For this review, take the finished solid that the model builds, in its own axes (mm). Face numbers are marked on the shaded views. A direction names the side the tool comes from. Round coordinates to 2 decimals unless told otherwise and drop trailing zeros. Loops run counter-clockwise (first coordinate to the right, second up) from the corner with the lowest first, then second, coordinate; pieces in that order, holes last.
1. To check wall thickness, follow line 1 along Z through (x, y) = (25.45, 0); line 2 along X through (y, z) = (7.75, 17.5); line 3 along Z through (x, y) = (0.5, 8.5). State the ranges of each line that lie inside material, in increasing order.
2. Consider section C-C on y = 10. State the section outline as (x, z) points, then the cut area to 3 significant figures.
3. Tool access review of the marked faces 1, 2 and 3: name each direction out of +Z, -Z, +X, -X, +Y, -Y from which nothing blocks a thin tool from reaching the whole face with its end or side.
4. Consider section D-D on y = -7.25. State the section outline as (x, z) points, then the cut area to 3 significant figures.
5. Clearance check with flat-ended pins moving along their axes: pin 1 Ø1.2 at (y, z) = (14, 10) entering from +X; pin 2 Ø4 at (y, z) = (3, 5) entering from -X; pin 3 Ø4 at (x, y) = (-2.5, 8.5) entering from +Z. State where each tip first meets the part, or that it passes through.
6. Consider section B-B on z = 3. State the section outline as (x, y) points, then the cut area to 3 significant figures.
7. Consider section A-A on y = 0. State the section outline as (x, z) points, then the cut area to 3 significant figures.
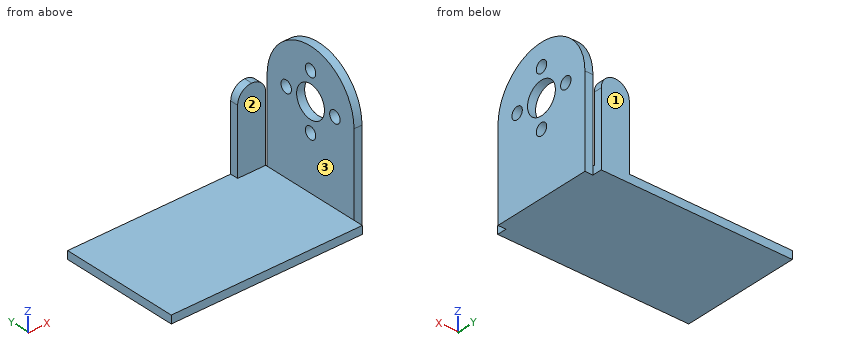
from build123d import *

# Parameters (mm, degrees)
SKETCH_1_W          = 47.7
SKETCH_1_H          = 29.8
EXTRUDE_1_DEPTH     = 2
SKETCH_2_W          = 7
SKETCH_2_H          = 2
EXTRUDE_3_DEPTH     = 19.9
CUT_EXTRUDE_1_DEPTH = 43.676369339
SKETCH_4_R          = 4
SKETCH_4_R_2        = 1.5
EXTRUDE_4_DEPTH     = 2
SKETCH_5_R          = 4
SKETCH_5_R_2        = 1.5
EXTRUDE_5_DEPTH     = 2


with BuildPart() as part:
    # 스케치1 → 보스-돌출1 (new body)
    with BuildSketch(Plane.XY):
        Rectangle(SKETCH_1_W, SKETCH_1_H)
    extrude(amount=EXTRUDE_1_DEPTH)

    # 스케치2 → 보스-돌출3 (add)
    with BuildSketch(Plane.XY.offset(2)):
        with Locations((20.35, 13.9)):
            Rectangle(SKETCH_2_W, SKETCH_2_H)
    extrude(amount=EXTRUDE_3_DEPTH)

    # 스케치3 → 컷-돌출1 (cut, through all)
    with BuildSketch(Plane.XZ.offset(-12.9)):
        with BuildLine():
            Line((16.85, 21.9), (16.85, 18.4))
            ThreePointArc((16.85, 18.4), (17.875126266, 20.874873734), (20.35, 21.9))
            Line((20.35, 21.9), (16.85, 21.9))
        make_face()
        with BuildLine():
            ThreePointArc((20.35, 21.9), (22.824873734, 20.874873734), (23.85, 18.4))
            Line((23.85, 18.4), (23.85, 21.9))
            Line((23.85, 21.9), (20.35, 21.9))
        make_face()
    extrude(amount=-CUT_EXTRUDE_1_DEPTH, mode=Mode.SUBTRACT)

    # 스케치4 → 보스-돌출4 (add)
    with BuildSketch(Plane(origin=(23.85, 0, 0), x_dir=(0, 0, -1), z_dir=(1, 0, 0))):
        with BuildLine():
            Line((0, 12.5), (0, -12.5))
            Line((0, -12.5), (-22.5, -12.5))
            ThreePointArc((-22.5, -12.5), (-35, 0), (-22.5, 12.5))
            Line((-22.5, 12.5), (0, 12.5))
        make_face()
        with Locations(Location((-22.5, 0, 0), (0, 0, 90))):
            Circle(SKETCH_4_R, mode=Mode.SUBTRACT)
        with Locations(Location((-29.5, 0, 0), (0, 0, 90))):
            Circle(SKETCH_4_R_2, mode=Mode.SUBTRACT)
        with Locations(Location((-22.5, 7, 0), (0, 0, 90))):
            Circle(SKETCH_4_R_2, mode=Mode.SUBTRACT)
        with Locations(Location((-15.5, 0, 0), (0, 0, 90))):
            Circle(SKETCH_4_R_2, mode=Mode.SUBTRACT)
        with Locations(Location((-22.5, -7, 0), (0, 0, 90))):
            Circle(SKETCH_4_R_2, mode=Mode.SUBTRACT)
    extrude(amount=EXTRUDE_4_DEPTH)

    # 스케치5 → 보스-돌출5 (add)
    with BuildSketch(Plane(origin=(23.85, 0, 0), x_dir=(0, 0, -1), z_dir=(1, 0, 0))):
        with BuildLine():
            Line((0, 12.5), (-22.5, 12.5))
            ThreePointArc((-22.5, 12.5), (-35, 0), (-22.5, -12.5))
            Line((-22.5, -12.5), (0, -12.5))
            Line((0, -12.5), (0, 12.5))
        make_face()
        with Locations(Location((-22.5, 0, 0), (0, 0, 90))):
            Circle(SKETCH_5_R, mode=Mode.SUBTRACT)
        with Locations(Location((-15.5, 0, 0), (0, 0, 90))):
            Circle(SKETCH_5_R_2, mode=Mode.SUBTRACT)
        with Locations(Location((-22.5, -7, 0), (0, 0, 90))):
            Circle(SKETCH_5_R_2, mode=Mode.SUBTRACT)
        with Locations(Location((-29.5, 0, 0), (0, 0, 90))):
            Circle(SKETCH_5_R_2, mode=Mode.SUBTRACT)
        with Locations(Location((-22.5, 7, 0), (0, 0, 90))):
            Circle(SKETCH_5_R_2, mode=Mode.SUBTRACT)
    extrude(amount=EXTRUDE_5_DEPTH)


solid = part.part
Resolved:
1. line 1: z = 0 to 14, 17 to 18.5, 26.5 to 28, 31 to 35
1. line 2: x = 23.85 to 25.85
1. line 3: z = 0 to 2
2. outline: (-23.85, 0) - (25.85, 0) - (25.85, 30) - (23.85, 30) - (23.85, 2) - (-23.85, 2) - close
2. area: 155 mm2
3. face 1: +Z, -Z, +X, -X, +Y
3. face 2: +Z, +X, -X, -Y
3. face 3: +Z, -X, -Y
4. outline: (-23.85, 0) - (25.85, 0) - (25.85, 21.02) - (23.85, 21.02) - (23.85, 2) - (-23.85, 2) - close; (23.85, 23.98) - (25.85, 23.98) - (25.85, 32.68) - (23.85, 32.68) - close
4. area: 155 mm2
5. pin 1: stops at x = 23.85
5. pin 2: stops at x = 23.85
5. pin 3: stops at z = 2
6. outline: (16.85, 12.9) - (23.85, 12.9) - (23.85, 14.9) - (16.85, 14.9) - close; (23.85, -12.5) - (25.85, -12.5) - (25.85, 12.5) - (23.85, 12.5) - close
6. area: 64.0 mm2
7. outline: (-23.85, 0) - (25.85, 0) - (25.85, 14) - (23.85, 14) - (23.85, 2) - (-23.85, 2) - close; (23.85, 17) - (25.85, 17) - (25.85, 18.5) - (23.85, 18.5) - close; (23.85, 26.5) - (25.85, 26.5) - (25.85, 28) - (23.85, 28) - close; (23.85, 31) - (25.85, 31) - (25.85, 35) - (23.85, 35) - close
7. area: 137 mm2
